```python
from build123d import *

# Parameters (mm, degrees)
SKETCH1_W           = 62.5
SKETCH1_H           = 25.4
BOSS_EXTRUDE1_DEPTH = 3
FILLET1_R           = 3
SKETCH2_R           = 1.75
CUT_EXTRUDE1_DEPTH  = 34.865210763
SKETCH6_W           = 6.5
SKETCH6_H           = 6.5
BOSS_EXTRUDE2_DEPTH = 2
SKETCH7_W           = 5
SKETCH7_H           = 10
BOSS_EXTRUDE3_DEPTH = 1.5


with BuildPart() as part:
    # Sketch1 → Boss-Extrude1 (new body)
    with BuildSketch(Plane(origin=(0, 0, 0), x_dir=(1, 0, 0), z_dir=(0, 1, 0))):
        Rectangle(SKETCH1_W, SKETCH1_H)
    extrude(amount=BOSS_EXTRUDE1_DEPTH)

    # Fillet1
    fillet1_edges = [part.edges().sort_by_distance(p)[0] for p in [
        (31.25, 1.5, 12.7),
        (-31.25, 1.5, 12.7),
        (-31.25, 1.5, -12.7),
        (31.25, 1.5, -12.7),
    ]]
    fillet(fillet1_edges, radius=FILLET1_R)

    # Sketch2 → Cut-Extrude1 (cut, through all)
    with BuildSketch(Plane(origin=(0, 3, 0), x_dir=(1, 0, 0), z_dir=(0, 1, 0))):
        with Locations(Location((-28, 9, 0), (0, 0, 270))):
            Circle(SKETCH2_R)
        with Locations(Location((28, 9, 0), (0, 0, 270))):
            Circle(SKETCH2_R)
        with Locations(Location((28, -9, 0), (0, 0, 270))):
            Circle(SKETCH2_R)
        with Locations(Location((-28, -9, 0), (0, 0, 270))):
            Circle(SKETCH2_R)
    extrude(amount=-CUT_EXTRUDE1_DEPTH, mode=Mode.SUBTRACT)

    # Sketch6 → Boss-Extrude2 (add)
    with BuildSketch(Plane(origin=(0, 3, 0), x_dir=(1, 0, 0), z_dir=(0, 1, 0))):
        with Locations((-7.25, 8.45)):
            Rectangle(SKETCH6_W, SKETCH6_H)
    extrude(amount=BOSS_EXTRUDE2_DEPTH)

    # Sketch7 → Boss-Extrude3 (add)
    with BuildSketch(Plane(origin=(0, 3, 0), x_dir=(1, 0, 0), z_dir=(0, 1, 0))):
        with Locations((4.5, 0)):
            Rectangle(SKETCH7_W, SKETCH7_H)
    extrude(amount=BOSS_EXTRUDE3_DEPTH)


solid = part.part
```
Verification items for the finished model (mm, model axes). A direction names the side the tool comes from. Coordinates: 2 decimals unless noted, no trailing zeros. Loops run counter-clockwise (first coordinate to the right, second up) from the corner with the lowest first, then second, coordinate; pieces in that order, holes last. Notation, with made-up numbers: (-22, -5.75) - (10, -5.75) arc R20 ccw to (10, 10.25) - close; hole circle Ø4 at (-30.5, 0.5). An arc over 180 degrees is marked (long way). Return JSON: item names as keys, results as strings.
1. Section check B-B, the plane y = 1.05. Record the boundary of the cut face in (x, z), then the cut area to 3 significant figures.
Established:
{"outline": "(-31.25, -9.7) arc R3 ccw to (-28.25, -12.7) - (28.25, -12.7) arc R3 ccw to (31.25, -9.7) - (31.25, 9.7) arc R3 ccw to (28.25, 12.7) - (-28.25, 12.7) arc R3 ccw to (-31.25, 9.7) - close; hole circle Ø3.5 at (-28, -9); hole circle Ø3.5 at (-28, 9); hole circle Ø3.5 at (28, -9); hole circle Ø3.5 at (28, 9)", "area": "1,540 mm2"}
2. Section check A-A, the plane z = -9. Record the boundary of the cut face in (x, y).
Established:
{"outline": "(-31.25, 0) - (-29.75, 0) - (-29.75, 3) - (-31.25, 3) - close; (-26.25, 0) - (26.25, 0) - (26.25, 3) - (-4, 3) - (-4, 5) - (-10.5, 5) - (-10.5, 3) - (-26.25, 3) - close; (29.75, 0) - (31.25, 0) - (31.25, 3) - (29.75, 3) - close"}
3. Mould release check, pull along X, two halves, no side actions. Record for faces 5 (the cylindrical face through (-30.39, 1.52, 11.8)), 6 (the cylindrical face through (-26.5, 1.5, -8.1)), 7 (the flat face through (4, 4, -5)), 8 (the cylindrical face through (30.39, 1.52, -11.8)): +X half, -X half, draft (parallel to the pull), parting line (faces both ways), or undercut.
Established:
{"face 5": "-X half", "face 6": "undercut", "face 7": "draft", "face 8": "+X half"}
4. Go/stop test with flat-tipped pins: pin 1 (3 mm diameter, centred on x = -11, z = -1, fed in from -Y); pin 2 (1.6 mm diameter, centred on x = -8, y = 4.5, fed in from -Z); pin 3 (1.2 mm diameter, centred on y = 4, z = 1.5, fed in from +X); pin 4 (2 mm diameter, centred on x = 28, z = 9, fed in from +Y). Record where each tip stops, or that it passes through.
Established:
{"pin 1": "stops at y = 0", "pin 2": "stops at z = -11.7", "pin 3": "stops at x = 7", "pin 4": "passes through"}
5. Section check D-D, the plane z = -2.5. Record the boundary of the cut face in (x, y).
Established:
{"outline": "(-31.25, 0) - (31.25, 0) - (31.25, 3) - (7, 3) - (7, 4.5) - (2, 4.5) - (2, 3) - (-31.25, 3) - close"}
6. Section check C-C, the plane x = -27. Record the boundary of the cut face in (y, z).
Established:
{"outline": "(0, -12.7) - (3, -12.7) - (3, -10.44) - (0, -10.44) - close; (0, -7.56) - (3, -7.56) - (3, 7.56) - (0, 7.56) - close; (0, 10.44) - (3, 10.44) - (3, 12.7) - (0, 12.7) - close"}
7. Thickness scan on L1, parallel to X at y = 1.85, z = -9; L2, parallel to X at y = 3.6, z = 3.25; L3, parallel to Y at x = -27, z = -5.75. Record the ranges inside material, lowest first.
Established:
{"L1": "x = -31.25 to -29.75, -26.25 to 26.25, 29.75 to 31.25", "L2": "x = 2 to 7", "L3": "y = 0 to 3"}
8. Tool access check on faces 1 (the flat face through (-7, 4, -11.7)), 2 (the cylindrical face through (-26.5, 1.5, 9.9)), 3 (the flat face through (4, 4, 5)), 4 (the flat face through (-10.5, 4, -8)). Record the directions out of +Z, -Z, +X, -X, +Y, -Y that give a thin tool (end or side, any length) a straight path to the whole face; none if there is none.
Established:
{"face 1": "-Z, +X, -X, +Y", "face 2": "+Y, -Y", "face 3": "+Z, +X, -X, +Y", "face 4": "+Z, -Z, -X, +Y"}
